```python
from build123d import *

# Parameters (mm, degrees)
SKETCH001_R        = 3.1
SKETCH001_R_2      = 1
PAD_DEPTH          = 5
SKETCH_W           = 73
SKETCH_H           = 64
SKETCH_W_2         = 43
SKETCH_H_2         = 34
PAD001_DEPTH       = 3
POLARPATTERN_COUNT = 2
FILLET_R           = 2
FILLET001_R        = 1
FILLET002_R        = 1
FILLET003_R        = 1
FILLET004_R        = 1


with BuildPart() as part:
    # Sketch001 → Pad (new body)
    with BuildSketch(Plane.XY.offset(3)):
        with Locations((-29, 24.5)):
            Circle(SKETCH001_R)
        with Locations((-29, 24.5)):
            Circle(SKETCH001_R_2, mode=Mode.SUBTRACT)
    pad = extrude(amount=PAD_DEPTH)

    # Sketch → Pad001 (join)
    with BuildSketch(Plane.XY):
        Rectangle(SKETCH_W, SKETCH_H)
        Rectangle(SKETCH_W_2, SKETCH_H_2, mode=Mode.SUBTRACT)
    extrude(amount=PAD001_DEPTH)

    # Mirrored: Pad across Sketch001 V_Axis
    add(pad.mirror(Plane(origin=(0, 0, 3), x_dir=(0, 0, 1), z_dir=(1, 0, 0))))

    # PolarPattern: Pad ×2 about axis
    polarpattern_axis = Axis((0, 0, 3), (0, 0, 1))
    for i in range(1, POLARPATTERN_COUNT):
        add(pad.rotate(polarpattern_axis, i * 360 / POLARPATTERN_COUNT))

    # Mirrored001: Pad across XZ
    add(pad.mirror(Plane.XZ))

    # Fillet
    fillet_edges = [part.edges().sort_by_distance(p)[0] for p in [
        (0, 32, 3),
        (-36.5, 0, 3),
        (36.5, 0, 3),
        (0, -32, 3),
        (-32.1, -24.5, 3),
        (32.1, -24.5, 3),
        (-32.1, 24.5, 3),
        (0, 17, 3),
        (-21.5, 0, 3),
        (21.5, 0, 3),
        (0, -17, 3),
        (32.1, 24.5, 3),
    ]]
    fillet(fillet_edges, radius=FILLET_R)

    # Fillet001
    fillet001_edges = [part.edges().sort_by_distance(p)[0] for p in [
        (-36.5, -32, 0.5),
    ]]
    fillet(fillet001_edges, radius=FILLET001_R)

    # Fillet002
    fillet002_edges = [part.edges().sort_by_distance(p)[0] for p in [
        (-36.5, 32, 0.5),
    ]]
    fillet(fillet002_edges, radius=FILLET002_R)

    # Fillet003
    fillet003_edges = [part.edges().sort_by_distance(p)[0] for p in [
        (36.5, 32, 0.5),
    ]]
    fillet(fillet003_edges, radius=FILLET003_R)

    # Fillet004
    fillet004_edges = [part.edges().sort_by_distance(p)[0] for p in [
        (36.5, -32, 0.5),
    ]]
    fillet(fillet004_edges, radius=FILLET004_R)


solid = part.part
```
The model under review builds one solid part; all positions refer to its coordinate system, in mm. A direction names the side the tool comes from. Give positions to 0.01 mm unless a question says otherwise; leave off trailing zeros. Write each loop counter-clockwise with the first axis right and the second up, starting at its lowest first coordinate (ties: lowest second). Pieces come first, ordered by that corner, then holes.
(1) Consider section D-D, the plane x = -29. Give the boundary of the cut face in (y, z), and give its area (3 significant figures).
(2) Consider section B-B, the plane y = -3. Give the boundary of the cut face in (x, z).
(3) To check wall thickness, follow L1, parallel to Y at x = -29, z = 7.05; L2, parallel to X at y = -24.5, z = 5.6; L3, parallel to Z at x = 28.5, y = -9. State the ranges of each line that lie inside material, in increasing order.
(4) For P1, Ø1.6, axis at x = 29, y = -24.5, coming from the +Z side; P2, Ø1, axis at x = -23.5, z = 2.5, coming from the -Y side; P3, Ø1.5, axis at x = 17, z = 3.5, coming from the -Y side, all flat-tipped, find the tip position at first contact; note any pin that passes through.
(5) The part is to be moulded in two halves that separate along Y. For faces 3 (the cylindrical face through (0.5, -31.43, 2.4)), 4 (the cylindrical face through (0.5, 31.43, 2.4)), 5 (the flat face through (29, -24, 3)), 6 (the flat face through (-29, 23, 8)), say which applies: released by +Y, released by -Y, zero draft, split by the parting line, or undercut.
(6) Tool access review of faces 1 (the cylindrical face through (32.1, 24.6, 6.5)), 2 (the cylindrical face through (-35.93, 0.43, 2.4)): name each direction out of +Z, -Z, +X, -X, +Y, -Y from which nothing blocks a thin tool from reaching the whole face with its end or side.
(7) Consider section C-C, the plane x = -20.5. Give the boundary of the cut face in (y, z).
(8) Consider section A-A, the plane z = 7. Give the boundary of the cut face in (x, y).
Returned:
1. outline: (-32, 0) - (32, 0) - (32, 1) arc R2 ccw to (30, 3) - (29.6, 3) arc R2 cw to (27.6, 5) - (27.6, 8) - (25.5, 8) - (25.5, 3) - (23.5, 3) - (23.5, 8) - (21.4, 8) - (21.4, 5) arc R2 cw to (19.4, 3) - (-19.4, 3) arc R2 cw to (-21.4, 5) - (-21.4, 8) - (-23.5, 8) - (-23.5, 3) - (-25.5, 3) - (-25.5, 8) - (-27.6, 8) - (-27.6, 5) arc R2 cw to (-29.6, 3) - (-30, 3) arc R2 ccw to (-32, 1) - close
1. area: 236 mm2
2. outline: (-36.5, 0) - (-21.5, 0) - (-21.5, 1) arc R2 ccw to (-23.5, 3) - (-34.5, 3) arc R2 ccw to (-36.5, 1) - close; (21.5, 0) - (36.5, 0) - (36.5, 1) arc R2 ccw to (34.5, 3) - (23.5, 3) arc R2 ccw to (21.5, 1) - close
3. L1: y = -27.6 to -25.5, -23.5 to -21.4, 21.4 to 23.5, 25.5 to 27.6
3. L2: x = -32.1 to -30, -28 to -25.9, 25.9 to 28, 30 to 32.1
3. L3: z = 0 to 3
4. P1: stops at z = 3
4. P2: stops at y = -31.73
4. P3: stops at y = -30.97
5. face 3: released by -Y
5. face 4: released by +Y
5. face 5: undercut
5. face 6: zero draft
6. face 1: +Z
6. face 2: +Z, -X, +Y, -Y
7. outline: (-32, 0) - (-17, 0) - (-17, 1) arc R2 ccw to (-19, 3) - (-30, 3) arc R2 ccw to (-32, 1) - close; (17, 0) - (32, 0) - (32, 1) arc R2 ccw to (30, 3) - (19, 3) arc R2 ccw to (17, 1) - close
8. outline: circle Ø6.2 at (-29, -24.5); circle Ø6.2 at (-29, 24.5); circle Ø6.2 at (29, -24.5); circle Ø6.2 at (29, 24.5); hole circle Ø2 at (-29, -24.5); hole circle Ø2 at (-29, 24.5); hole circle Ø2 at (29, -24.5); hole circle Ø2 at (29, 24.5)
